Read the model definition and answer for the solid it produces. Units are mm, in the model's axes. Face numbers are marked on the shaded views. A direction names the side the tool comes from. Coordinates: 2 decimals unless noted, no trailing zeros. Order: outer loops, then holes, each group sorted by start corner. A loop starts at its lowest first (then second) coordinate and runs counter-clockwise, first axis right, second up. Notation, with made-up numbers: (-31, -7) -> (15, -7) arc R14 cw to (15, 10) -> close; hole circle Ø9 at (52.5, -34). An arc over 180 degrees is marked (long way). Use CSV: the item, a comma, the result in double quotes.
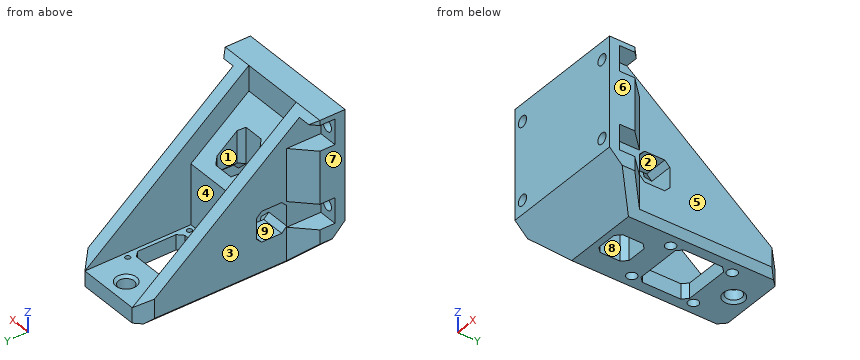
```python
from build123d import *

# Parameters (mm, degrees)
SKETCH1_W               = 50
SKETCH1_H               = 58.25
BOSS_EXTRUDE1_DEPTH     = 10
SKETCH2_R               = 2.15
CUT_EXTRUDE1_DEPTH      = 4
SKETCH5_W               = 25
SKETCH5_H               = 6
BOSS_EXTRUDE3_DEPTH     = 65
CUT_EXTRUDE3_REACH      = 100.199
SKETCH6_W               = 22
SKETCH6_H               = 19.25
SKETCH7_R               = 1
CUT_EXTRUDE4_DEPTH      = 2.5
CUT_EXTRUDE5_REACH      = 98.164
SKETCH8_R               = 2
BOSS_EXTRUDE4_DEPTH     = 5
CHAMFER1_SIZE           = 7.5
CHAMFER2_SIZE           = 10
CHAMFER4_SIZE           = 15
CHAMFER5_SIZE           = 5
CHAMFER7_SIZE           = 2
CUT_EXTRUDE6_REACH      = 100.199
SKETCH10_R              = 3.1
CHAMFER8_SIZE           = 1
BOSS_EXTRUDE5_REACH     = 90.767
CUT_EXTRUDE7_REACH      = 100.199
SKETCH12_W              = 12
SKETCH12_H              = 12
CUT_EXTRUDE9_REACH      = 88.222
SKETCH14_W              = 12
SKETCH14_H              = 12
CHAMFER11_SIZE          = 2
CUT_EXTRUDE12_OUTLINE_W = 10
CUT_EXTRUDE12_OUTLINE_H = 13.5
CUT_EXTRUDE12_DEPTH     = 7.5
LPATTERN1_COUNT         = 2
LPATTERN1_PITCH         = 30.7
MIRROR3_COPY_1_SKETCH_W = 10
MIRROR3_COPY_1_SKETCH_H = 13.5
MIRROR3_COPY_1_DEPTH    = 7.5


# Read off the part's stored shape, not the designer's step: Cut-Extrude12
with BuildPart() as part:
    # Sketch1 → Boss-Extrude1 (new body)
    with BuildSketch(Plane(origin=(0, 0, 0), x_dir=(1, 0, 0), z_dir=(0, 1, 0))):
        Rectangle(SKETCH1_W, SKETCH1_H)
    extrude(amount=BOSS_EXTRUDE1_DEPTH)

    # Sketch2 → Cut-Extrude1 (cut)
    with BuildSketch(Plane(origin=(0, 0, 0), x_dir=(1, 0, 0), z_dir=(0, 1, 0))):
        with Locations(Location((-21, 8.575, 0), (0, 0, 270))):
            Circle(SKETCH2_R)
        with Locations(Location((-21, -22.125, 0), (0, 0, 270))):
            Circle(SKETCH2_R)
        with Locations(Location((21, 8.575, 0), (0, 0, 270))):
            Circle(SKETCH2_R)
        with Locations(Location((21, -22.125, 0), (0, 0, 270))):
            Circle(SKETCH2_R)
    extrude(amount=CUT_EXTRUDE1_DEPTH, mode=Mode.SUBTRACT)

    # Sketch5 → Boss-Extrude3 (add)
    with BuildSketch(Plane(origin=(0, 10, 0), x_dir=(1, 0, 0), z_dir=(0, 1, 0))):
        with Locations((0, 26.125)):
            Rectangle(SKETCH5_W, SKETCH5_H)
    extrude(amount=BOSS_EXTRUDE3_DEPTH)

    # Sketch6 → Cut-Extrude3 (cut, up to next)
    with BuildSketch(Plane(origin=(0, 0, -29.125), x_dir=(-1, 0, 0), z_dir=(0, 0, -1)), mode=Mode.PRIVATE) as cut_extrude3_sk1:
        with Locations((0, 47.625)):
            Rectangle(SKETCH6_W, SKETCH6_H)
    cut_extrude3_tool1 = extrude(cut_extrude3_sk1.sketch, amount=-CUT_EXTRUDE3_REACH, mode=Mode.PRIVATE) & part.part
    add(cut_extrude3_tool1.solids().sort_by_distance((0, 47.625, -29.125))[0], mode=Mode.SUBTRACT)

    # Sketch7 → Cut-Extrude4 (cut)
    with BuildSketch(Plane.XY.offset(-23.125)):
        with Locations((10.25, 35.25)):
            Circle(SKETCH7_R)
        with Locations((-10.25, 35.25)):
            Circle(SKETCH7_R)
        with Locations((-10.25, 59.7)):
            Circle(SKETCH7_R)
        with Locations((10.25, 59.7)):
            Circle(SKETCH7_R)
    extrude(amount=-CUT_EXTRUDE4_DEPTH, mode=Mode.SUBTRACT)

    # Sketch8 → Cut-Extrude5 (cut, up to next)
    with BuildSketch(Plane.XY.offset(-25.625), mode=Mode.PRIVATE) as cut_extrude5_sk1:
        with Locations((-10.25, 59.7)):
            Circle(SKETCH8_R)
    cut_extrude5_tool1 = extrude(cut_extrude5_sk1.sketch, amount=-CUT_EXTRUDE5_REACH, mode=Mode.PRIVATE) & part.part
    # Sketch8 → Cut-Extrude5 (cut, up to next)
    with BuildSketch(Plane.XY.offset(-25.625), mode=Mode.PRIVATE) as cut_extrude5_sk2:
        with Locations((10.25, 59.7)):
            Circle(SKETCH8_R)
    cut_extrude5_tool2 = extrude(cut_extrude5_sk2.sketch, amount=-CUT_EXTRUDE5_REACH, mode=Mode.PRIVATE) & part.part
    # Sketch8 → Cut-Extrude5 (cut, up to next)
    with BuildSketch(Plane.XY.offset(-25.625), mode=Mode.PRIVATE) as cut_extrude5_sk3:
        with Locations((10.25, 35.25)):
            Circle(SKETCH8_R)
    cut_extrude5_tool3 = extrude(cut_extrude5_sk3.sketch, amount=-CUT_EXTRUDE5_REACH, mode=Mode.PRIVATE) & part.part
    # Sketch8 → Cut-Extrude5 (cut, up to next)
    with BuildSketch(Plane.XY.offset(-25.625), mode=Mode.PRIVATE) as cut_extrude5_sk4:
        with Locations((-10.25, 35.25)):
            Circle(SKETCH8_R)
    cut_extrude5_tool4 = extrude(cut_extrude5_sk4.sketch, amount=-CUT_EXTRUDE5_REACH, mode=Mode.PRIVATE) & part.part
    add(cut_extrude5_tool1.solids().sort_by_distance((-10.25, 59.7, -25.625))[0], mode=Mode.SUBTRACT)
    add(cut_extrude5_tool2.solids().sort_by_distance((10.25, 59.7, -25.625))[0], mode=Mode.SUBTRACT)
    add(cut_extrude5_tool3.solids().sort_by_distance((10.25, 35.25, -25.625))[0], mode=Mode.SUBTRACT)
    add(cut_extrude5_tool4.solids().sort_by_distance((-10.25, 35.25, -25.625))[0], mode=Mode.SUBTRACT)

    # Sketch9 → Boss-Extrude4 (add)
    with BuildSketch(Plane(origin=(12.5, 0, 0), x_dir=(0, 0, -1), z_dir=(1, 0, 0))):
        Polygon((29.125, 75), (23.125, 75), (-29.125, 10), (29.125, 10), align=None)
    boss_extrude4 = extrude(amount=BOSS_EXTRUDE4_DEPTH)

    # Mirror1: Boss-Extrude4 across plane
    add(boss_extrude4.mirror(Plane(origin=(0, 0, 0), x_dir=(0, 0, 1), z_dir=(1, 0, 0))))

    # Chamfer1
    chamfer1_edges = [part.edges().sort_by_distance(p)[0] for p in [
        (17.5, 10, 0),
        (-17.5, 10, 0),
    ]]
    chamfer(chamfer1_edges, length=CHAMFER1_SIZE - 0.0001)  # a hair under: the kernel refuses the full size

    # Chamfer2
    chamfer2_edges = [part.edges().sort_by_distance(p)[0] for p in [
        (-25, 5, -29.125),
        (25, 5, -29.125),
    ]]
    chamfer(chamfer2_edges, length=CHAMFER2_SIZE)

    # Chamfer4
    chamfer4_edges = [part.edges().sort_by_distance(p)[0] for p in [
        (0, 0, -29.125),
    ]]
    chamfer(chamfer4_edges, length=CHAMFER4_SIZE)

    # Chamfer5
    chamfer5_edges = [part.edges().sort_by_distance(p)[0] for p in [
        (17.5, 75, -24.875),
        (-17.5, 75, -24.875),
    ]]
    chamfer(chamfer5_edges, length=CHAMFER5_SIZE)

    # Chamfer7
    chamfer7_edges = [part.edges().sort_by_distance(p)[0] for p in [
        (-11, 57.25, -26.125),
        (-11, 38, -26.125),
        (11, 38, -26.125),
        (11, 57.25, -26.125),
    ]]
    chamfer(chamfer7_edges, length=CHAMFER7_SIZE)

    # Sketch10 → Cut-Extrude6 (cut, up to next)
    with BuildSketch(Plane(origin=(0, 0, -29.125), x_dir=(-1, 0, 0), z_dir=(0, 0, -1)), mode=Mode.PRIVATE) as cut_extrude6_sk1:
        with Locations((0, 68)):
            Circle(SKETCH10_R)
    cut_extrude6_tool1 = extrude(cut_extrude6_sk1.sketch, amount=-CUT_EXTRUDE6_REACH, mode=Mode.PRIVATE) & part.part
    add(cut_extrude6_tool1.solids().sort_by_distance((0, 68, -29.125))[0], mode=Mode.SUBTRACT)

    # Chamfer8
    chamfer8_edges = [part.edges().sort_by_distance(p)[0] for p in [
        (3.1, 68, -29.125),
        (3.1, 68, -23.125),
    ]]
    chamfer(chamfer8_edges, length=CHAMFER8_SIZE)

    # Sketch11 → Boss-Extrude5 (add, up to next)
    with BuildSketch(Plane(origin=(-12.5, 0, 0), x_dir=(0, 0, -1), z_dir=(1, 0, 0)), mode=Mode.PRIVATE) as boss_extrude5_sk1:
        Polygon((-19.125, 10), (23.125, 10), (23.125, 33), (-0.636538462, 33), align=None)
    boss_extrude5_tool1 = extrude(boss_extrude5_sk1.sketch, amount=BOSS_EXTRUDE5_REACH, mode=Mode.PRIVATE) - part.part
    add(boss_extrude5_tool1.solids().sort_by_distance((-12.5, 20.426363, -6.190596))[0])

    # Cut-Extrude7: up to this plane
    cut_extrude7_end = Plane(origin=(25.002, 33, 0.636538462), z_dir=(0, -0.6265212074854106, -0.7794043729483581))
    # Sketch12 → Cut-Extrude7 (cut, up to the surface)
    with BuildSketch(Plane(origin=(0, 0, -29.125), x_dir=(-1, 0, 0), z_dir=(0, 0, -1)), mode=Mode.PRIVATE) as cut_extrude7_sk1:
        with Locations((0, 23.5)):
            Rectangle(SKETCH12_W, SKETCH12_H)
    cut_extrude7_tool1 = split(extrude(cut_extrude7_sk1.sketch, amount=-CUT_EXTRUDE7_REACH, mode=Mode.PRIVATE), bisect_by=cut_extrude7_end, keep=Keep.BOTH, mode=Mode.PRIVATE)
    add(cut_extrude7_tool1.solids().sort_by_distance((0, 23.5, -29.125))[0], mode=Mode.SUBTRACT)

    # Sketch14 → Cut-Extrude9 (cut, up to next)
    with BuildSketch(Plane(origin=(-6, 0, 0), x_dir=(0, 0, -1), z_dir=(1, 0, 0)), mode=Mode.PRIVATE) as cut_extrude9_sk1:
        with Locations((9.125, 23.5)):
            Rectangle(SKETCH14_W, SKETCH14_H)
    cut_extrude9_tool1 = extrude(cut_extrude9_sk1.sketch, amount=-CUT_EXTRUDE9_REACH, mode=Mode.PRIVATE) & part.part
    cut_extrude9 = cut_extrude9_tool1.solids().sort_by_distance((-6, 23.5, -9.125))[0]
    add(cut_extrude9, mode=Mode.SUBTRACT)

    # Mirror2: Cut-Extrude9 across plane
    add(cut_extrude9.mirror(Plane(origin=(0, 0, 0), x_dir=(0, 0, 1), z_dir=(1, 0, 0))), mode=Mode.SUBTRACT)

    # Chamfer11
    chamfer11_edges = [part.edges().sort_by_distance(p)[0] for p in [
        (-6, 17.5, 4.985576923),
        (6, 17.5, 4.985576923),
        (6, 29.5, 0.1625),
        (-6, 29.5, 0.1625),
        (-6, 17.5, -22.125),
        (-6, 29.5, -22.125),
        (-11.75, 17.5, -15.125),
        (-11.75, 29.5, -15.125),
        (-11.75, 17.5, -3.125),
        (-11.75, 29.5, -3.125),
        (-6, 23.5, -15.125),
        (-6, 23.5, -3.125),
        (6, 29.5, -22.125),
        (6, 17.5, -22.125),
        (11.75, 17.5, -3.125),
        (11.75, 17.5, -15.125),
        (6, 23.5, -15.125),
        (11.75, 29.5, -15.125),
        (11.75, 29.5, -3.125),
        (6, 23.5, -3.125),
    ]]
    chamfer(chamfer11_edges, length=CHAMFER11_SIZE)

    # Cut-Extrude12 outline → Cut-Extrude12 (cut)
    with BuildSketch(Plane(origin=(17.5, 0, 0), x_dir=(0, 0, -1), z_dir=(1, 0, 0))):
        with Locations((8.575, 10.75)):
            Rectangle(CUT_EXTRUDE12_OUTLINE_W, CUT_EXTRUDE12_OUTLINE_H)
    cut_extrude12 = extrude(amount=CUT_EXTRUDE12_DEPTH, mode=Mode.SUBTRACT)

    # LPattern1: Cut-Extrude12 ×2
    with Locations(*[(0, 0, i * LPATTERN1_PITCH) for i in range(1, LPATTERN1_COUNT)]):
        add(cut_extrude12, mode=Mode.SUBTRACT)

    # Mirror3: Cut-Extrude12 across plane
    add(cut_extrude12.mirror(Plane(origin=(0, 0, 0), x_dir=(0, 0, 1), z_dir=(1, 0, 0))), mode=Mode.SUBTRACT)

    # Mirror3 copy 1 sketch → Mirror3 copy 1 (cut)
    with BuildSketch(Plane(origin=(-17.5, 0, 30.7), x_dir=(0, 0, -1), z_dir=(-1, 0, 0))):
        with Locations((8.575, -10.75)):
            Rectangle(MIRROR3_COPY_1_SKETCH_W, MIRROR3_COPY_1_SKETCH_H)
    extrude(amount=MIRROR3_COPY_1_DEPTH, mode=Mode.SUBTRACT)


solid = part.part
```
Item 1: A tool of negligible diameter and unlimited length cuts with its end or side. For the marked faces 1, 2, 3, 4 and 5, from which of +Z, -Z, +X, -X, +Y, -Y can it reach the whole face along a straight path? Write none if from no direction.
Return value:
face 1,"+Z, -Z"
face 2,"+X, -X"
face 3,"-X, +Y"
face 4,"+Z, +Y"
face 5,"+X, +Y"
Item 2: The mould has two halves that part along X. Classify the marked faces 6, 7, 8 and 9: +X half, -X half, draft (parallel to the pull), parting line (faces both ways), or undercut.
Return value:
face 6,"+X half"
face 7,"-X half"
face 8,"undercut"
face 9,"draft"
Item 3: Each of these flat-tipped pins is pushed along its axis until it touches: P1, Ø4, axis at y = 24, z = 6.5, coming from the -X side; P2, Ø4, axis at y = 24.5, z = -24, coming from the +X side; P3, Ø9, axis at x = -13, y = 23.5, coming from the +Z side. Where does it stop, or does it pass through?
Return value:
P1,"stops at x = -17.5"
P2,"stops at x = 17.5"
P3,"stops at z = 21.89"
Item 4: Find section C-C, the plane x = 0. Give the vertices of the cut face in (y, z) (3 decimals).
Return value:
outline,"(0, -14.125) -> (15, -29.125) -> (17.5, -29.125) -> (17.5, 13.096) -> (10, 19.125) -> (10, 29.125) -> (0, 29.125) -> close; (29.5, -29.125) -> (38, -29.125) -> (38, -23.125) -> (33, -23.125) -> (33, 0.637) -> (29.5, 3.45) -> close; (57.25, -29.125) -> (63.9, -29.125) -> (64.9, -28.125) -> (64.9, -24.125) -> (63.9, -23.125) -> (57.25, -23.125) -> close; (71.1, -28.125) -> (72.1, -29.125) -> (75, -29.125) -> (75, -23.125) -> (72.1, -23.125) -> (71.1, -24.125) -> close"
Item 5: Find section A-A, the plane x = -7. Give the vertices of the cut face in (y, z) (3 decimals), then the cut area to 3 significant figures.
Return value:
outline,"(0, -14.125) -> (15, -29.125) -> (38, -29.125) -> (38, -23.125) -> (33, -23.125) -> (33, 0.637) -> (10, 19.125) -> (10, 29.125) -> (0, 29.125) -> close; (57.25, -29.125) -> (75, -29.125) -> (75, -23.125) -> (57.25, -23.125) -> close; hole (17.5, -14.125) -> (19.5, -16.125) -> (27.5, -16.125) -> (29.5, -14.125) -> (29.5, -4.125) -> (27.5, -2.125) -> (19.5, -2.125) -> (17.5, -4.125) -> close"
area,"1,340 mm^2"
Item 6: Straight lines are drawn through the part: line 1 along X through (y, z) = (21.5, 6.5); line 2 along X through (y, z) = (53, -5.5); line 3 along Y through (x, z) = (-5, -9). For each, find the intervals that lie inside material, in ascending order.
Return value:
line 1,"x = -17.5 to -6, 6 to 17.5"
line 2,"x = -17.5 to -12.5, 12.5 to 17.5"
line 3,"y = 0 to 17.5, 29.5 to 33"
Item 7: Find section B-B, the plane z = -12. Give the vertices of the cut face in (x, y), then the cut area to 3 significant figures.
Return value:
outline,"(-25, 0) -> (25, 0) -> (25, 4) -> (17.5, 4) -> (17.5, 17.5) -> (-17.5, 17.5) -> (-17.5, 4) -> (-25, 4) -> close; (-17.5, 29.5) -> (17.5, 29.5) -> (17.5, 61.16) -> (12.5, 61.16) -> (12.5, 33) -> (-12.5, 33) -> (-12.5, 61.16) -> (-17.5, 61.16) -> close"
area,"1,080 mm^2"
Item 8: Find section D-D, the plane y = 68. Give the vertices of the cut face in (x, z) (3 decimals).
Return value:
outline,"(-17.5, -26.625) -> (-15, -29.125) -> (-4.1, -29.125) -> (-3.1, -28.125) -> (-3.1, -24.125) -> (-4.1, -23.125) -> (-12.5, -23.125) -> (-12.5, -17.498) -> (-17.5, -17.498) -> close; (3.1, -28.125) -> (4.1, -29.125) -> (15, -29.125) -> (17.5, -26.625) -> (17.5, -17.498) -> (12.5, -17.498) -> (12.5, -23.125) -> (4.1, -23.125) -> (3.1, -24.125) -> close"
